Autodesk Fusion 360 part; units mm, degrees
sketch "Sketch1" plane through (0, 0, 0) normal (0, 1, 0) x (1, 0, 0)
  circle A0 centre (0, 0) radius 25
  dimension "d1" = 50
extrude "Extrude1" add sketch "Sketch1" along normal blind 25
sketch "Sketch2" plane through (0, 0, 0) normal (0, 1, 0) x (1, 0, 0)
  line L0 (37.5, -37.5) -> (-37.5, -37.5)
  line L1 (-37.5, -37.5) -> (-37.5, 37.5)
  line L2 (-37.5, 37.5) -> (37.5, 37.5)
  line L3 (37.5, 37.5) -> (37.5, -37.5)
  line L4 (37.5, -37.5) -> (-37.5, 37.5) construction
  line L5 (-37.5, -37.5) -> (37.5, 37.5) construction
  dimension "d4" = 75
  dimension "d5" = 75
extrude "Extrude2" add sketch "Sketch2" against normal blind 5
chamfer "Chamfer1" distance 10 angle 45 1 edges at (-23.3082, 25, 9.0404)
Design review of the part built by this model. Coordinates are the model's own, in mm. A direction names the side the tool comes from. Give positions to 0.01 mm unless a question says otherwise; leave off trailing zeros. Order: outer loops, then holes, each group sorted by start corner. A loop starts at its lowest first (then second) coordinate and runs counter-clockwise, first axis right, second up. Notation, with made-up numbers: (-9.75, -27.5) - (48.25, -27.5) arc R19 ccw to (48.25, -16.5) - close; hole circle Ø11 at (-22.5, 50.25). An arc over 180 degrees is marked (long way). Use a Markdown table: item, result. Add a question column.
(1) Add section B-B on x = 0. Give the boundary of the cut face in (y, z), then the cut area to 4 significant figures.
(2) Wall thickness on probe 1 along Y at (x, z) = (34.5, -16); probe 2 along X at (y, z) = (5.5, 1); probe 3 along Z at (x, y) = (-4, 11.5): over which ranges is each line inside the solid? List them lowest first. Write a range as [from, to].
(3) Add section C-C on y = 21. Give the boundary of the cut face in (x, z), then the cut area to 3 significant figures.
(4) Clearance check with flat-ended pins moving along their axes: P1, Ø6, axis at x = -2, y = 5, coming from the -Z side; P2, Ø8, axis at y = 19, z = 12.5, coming from the -X side; P3, Ø1, axis at y = 18, z = 9, coming from the -X side; P4, Ø8, axis at x = -13.5, y = 2.5, coming from the -Z side. State where each tip first meets the part, or that it passes through.
(5) Add section A-A on z = 0. Give the boundary of the cut face in (x, y), then the cut area to 4 significant figures.
(6) Machinability: for faces 1 (the face through (-1, 0, -26)), 2 (the face through (0, 25, 0)), which of the approach directions +Z, -Z, +X, -X, +Y, -Y give a long, thin tool a straight path to every point of the face, cutting with its end or side? Answer none if there is none.
(7) Add section D-D on y = 4. Give the boundary of the cut face in (x, z).
Report:
| question | item | result |
|---|---|---|
| 1 | outline | (-5, -37.5) - (0, -37.5) - (0, -25) - (15, -25) - (25, -15) - (25, 15) - (15, 25) - (0, 25) - (0, 37.5) - (-5, 37.5) - close |
| 1 | area | 1,525 mm² |
| 2 | probe 1 | y = [-5, 0] |
| 2 | probe 2 | x = [-24.98, 24.98] |
| 2 | probe 3 | z = [-24.68, 24.68] |
| 3 | outline | circle Ø38 at (0, 0) |
| 3 | area | 1,130 mm² |
| 4 | P1 | stops at z = -25 |
| 4 | P2 | stops at x = -22.13 |
| 4 | P3 | stops at x = -20.66 |
| 4 | P4 | stops at z = -37.5 |
| 5 | outline | (-37.5, -5) - (37.5, -5) - (37.5, 0) - (25, 0) - (25, 15) - (15, 25) - (-15, 25) - (-25, 15) - (-25, 0) - (-37.5, 0) - close |
| 5 | area | 1,525 mm² |
| 6 | face 1 | +Y |
| 6 | face 2 | +Z, -Z, +X, -X, +Y |
| 7 | outline | circle Ø50 at (0, 0) |
